Autodesk Inventor part; units mm, degrees
ref_plane "Work Plane1" through (0, 0, 50.8) normal (0, 0, 1) x (1, 0, 0)
ref_plane "YZ Plane" through (0, 0, 0) normal (1, 0, 0) x (0, 1, 0)
ref_plane "XZ Plane" through (0, 0, 0) normal (0, 1, 0) x (-1, 0, 0)
sketch "Sketch2" plane through (0, 0, 0) normal (0, 0, 1) x (1, 0, 0)
  line L0 (0, 0) -> (25.4, 0)
  line L1 (25.4, 0) -> (25.4, 5.588)
  line L2 (25.4, 5.588) -> (0, 5.588)
  line L3 (0, 5.588) -> (0, 0)
  arc A0 (25.4, 0) -> (25.4, 5.588) centre (25.4, 2.794) ccw
  dimension "d0" = 25.4
  dimension "d1" = 5.588
ref_plane "Work Plane1" through (0, 0, 50.8) normal (0, 0, 1) x (1, 0, 0)
sketch "Sketch3" plane through (0, 0, 50.8) normal (0, 0, 1) x (1, 0, 0)
  line L0 (0, 1.2065) -> (6.35, 1.2065)
  line L1 (6.35, 1.2065) -> (6.35, 4.3815)
  line L2 (6.35, 4.3815) -> (0, 4.3815)
  line L3 (0, 4.3815) -> (0, 1.2065)
  arc A0 (6.35, 1.2065) -> (6.35, 4.3815) centre (6.35, 2.794) ccw
  point P0 (0, 0)
  dimension "d3" = 6.35
  dimension "d4" = 3.175
  dimension "d5" = 1.2065
loft "Loft1" add profiles "Sketch2", "Sketch3"
sketch "Sketch4" plane through (0, 0, 0) normal (-1, 0, 0) x (0, 0, 1)
  line L0 (0, 5.588) -> (0, 0)
  line L1 (0, 0) -> (50.8, 1.2065)
  line L2 (50.8, 4.3815) -> (50.8, 1.2065)
  line L3 (0, 5.588) -> (50.8, 4.3815)
  line L4 (0, 5.588) -> (50.8, 4.3815)
  line L5 (44.45, 4.5323) -> (44.45, 1.0557)
  line L6 (50.8, 1.2065) -> (0, 0)
  dimension "d10" = 6.35
extrude "Extrusion1" add sketch "Sketch4" along normal blind 38.608 contours L3 L2 L1 L5
sketch "Sketch5" plane through (25.4, 5.588, 0) normal (0, 0, -1) x (-1, 0, 0)
  line L0 (25.4, 0) -> (25.4, -5.588)
  line L1 (0, 0) -> (25.4, 0)
  arc A0 (0, 0) -> (0, -5.588) centre (0, -2.794) ccw
  line L2 (25.4, -5.588) -> (0, -5.588)
  line L3 (25.4, 0) -> (25.4, -5.588)
  line L4 (25.4, 0) -> (36.1487, 0)
  line L5 (36.1487, 0) -> (36.1487, -5.5776)
  line L6 (36.1487, -5.5776) -> (25.4, -5.5776)
  line L7 (25.4, -5.5776) -> (25.4, 0)
  line L8 (-3.175, -0.1076) -> (-3.175, -7.007)
  line L9 (25.4, -5.588) -> (0, -5.588)
revolve "Revolution1" add sketch "Sketch5" angle 15 about axis through (28.575, 5.4804, 0) along (0, -1, 0)
sketch "Sketch7" plane through (-10.7487, 5.588, 0) normal (0, 1, 0) x (1, 0, 0)
  line L0 (0, 0) -> (10.7487, 0)
  line L1 (36.1487, 0) -> (10.7487, 0)
  arc A0 (36.2569, 0.8218) -> (36.1487, 0) centre (39.3237, 0) ccw
  line L2 (1.3399, 10.1777) -> (36.2569, 0.8218)
  arc A1 (1.3399, 10.1777) -> (0, 0) centre (39.3237, 0) ccw
  line L3 (10.7487, 0) -> (10.7487, -44.45)
  line L4 (10.7487, 0) -> (-2.0556, 0)
  line L5 (-2.0556, 0) -> (-2.0556, 10.6947)
  line L6 (-2.0556, 10.6947) -> (10.7487, 10.6947)
  line L7 (10.7487, 10.6947) -> (10.7487, 0)
extrude "Extrusion2" cut sketch "Sketch7" against normal blind 38.1 contours A1 L2 L7 L0 | L4 L5 L6 L7 L2 A1
sketch "Sketch8" plane through (0, 0.0104, -7.6566) normal (0.258819, 0, -0.9659258) x (-0.9659258, 0, -0.258819)
  line L0 (-29.583, 2.7836) -> (-24.8205, 2.7836)
  line L1 (-24.8205, 2.7836) -> (-8.9455, 2.7836)
  circle A0 centre (-24.8205, 2.7836) radius 1.27
  circle A1 centre (-8.9455, 2.7836) radius 1.27
  line L2 (-26.408, -0.0104) -> (0, -0.0104)
  point P0 (-1.9817, -0.0104)
  point P1 (0, 0)
  dimension "d17" = 4.7625
  dimension "d18" = 15.875
  dimension "d19" = 2.54
  dimension "d20" = 2.54
  dimension "d23" = 2.794
extrude "Extrusion4" cut sketch "Sketch8" against normal blind 12.7
sketch "Sketch9" plane through (0, 1.0557, 44.45) normal (0, 0, -1) x (-1, 0, 0)
  line L0 (0, 0) -> (0, 3.4766)
  line L1 (0, 0) -> (38.608, 0)
  line L2 (38.608, 3.4766) -> (38.608, 0)
  line L3 (0, 3.4766) -> (38.608, 3.4766)
  point P0 (0, -1.0557)
extrude "Extrusion5" cut sketch "Sketch9" against normal through all
sketch "Sketch10" plane through (0, 1.2065, 50.8) normal (-1, 0, 0) x (0, 0, 1)
  line L0 (0, 3.175) -> (0, 0)
  line L1 (0, 2.4765) -> (-6.35, 2.4765)
  line L2 (-6.35, 2.4765) -> (-6.35, 0.6985)
  line L3 (-6.35, 0.6985) -> (0, 0.6985)
  line L4 (0, 0.6985) -> (0, 2.4765)
  line L5 (-50.8, 4.3815) -> (0, 3.175) construction
  line L6 (0, 2.4765) -> (0, 3.175) construction
  line L7 (0, 3.175) -> (0, 0) construction
  line L8 (0, 0.6985) -> (0, 0) construction
  point P0 (-50.8, -1.2065)
  dimension "d28" = 1.778
  dimension "d29" = 6.35
extrude "Extrusion6" cut sketch "Sketch10" against normal through all
properties part number "DivePlanesStabilizingFins_Print1"
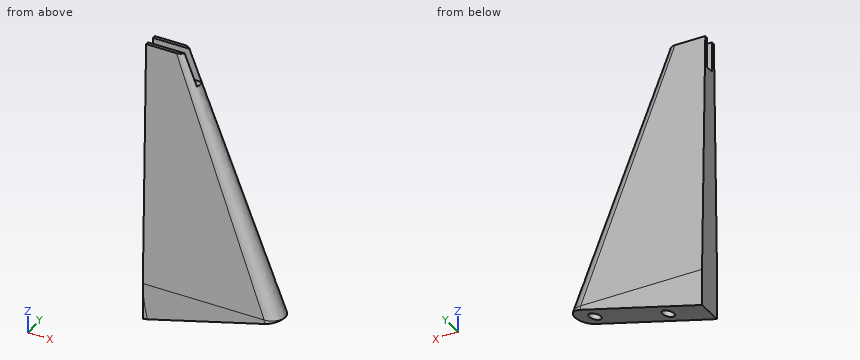
CAD build for the part. Positions are in the model's coordinates, mm. Round coordinates to 2 decimals unless told otherwise and drop trailing zeros.
(1) Slice it at B-B, the plane z = 5.5. Count the separate pieces of the cut face and the enclosed holes in it, and give its area (3 significant figures).
(2) Drop flat-ended pins along their axis: P1, Ø4, axis at x = 7.5, z = 3, coming from the +Y side; P2, Ø7, axis at x = 7.5, z = 46.5, coming from the -Y side; P3, Ø0.5, axis at x = 0.5, z = -4, coming from the -Y side; P4, Ø5, axis at x = 5, z = 48.5, coming from the +Y side. Give the stop position or say it passes through.
(3) Probe line 1 along X through (y, z) = (1.8, 5); line 2 along X through (y, z) = (2.35, 10); line 3 along Y through (x, z) = (9, -3.5). List the from-to ranges inside material, lowest first.
From the geometry:
1. separate pieces: 1
1. enclosed holes: 2
1. area: 125 mm2
2. P1: stops at y = 5.56
2. P2: stops at y = 1.02
2. P3: stops at y = 0
2. P4: stops at y = 4.5
3. line 1: x = 0 to 5.05, 6.69 to 21.49, 23.12 to 26.01
3. line 2: x = 0 to 19.73, 22.2 to 24.17
3. line 3: y = 0 to 1.83, 3.76 to 5.59
